Build history of the part. All positions in model axes, mm. Face numbers are marked on the shaded views. A direction names the side the tool comes from. Coordinates: 2 decimals unless noted, no trailing zeros. Loops run counter-clockwise (first coordinate to the right, second up) from the corner with the lowest first, then second, coordinate; pieces in that order, holes last.
Item 1: Cut at C-C (x = 109.5). List the corners of the cut face in (y, z).
Item 2: Drill centre lines: line 1 along X through (y, z) = (49, -20.5); line 2 along Z through (x, y) = (-56, 8.5); line 3 along X through (y, z) = (37, 3.5). Where is each one in solid material? Low to high.
Item 3: 3-axis set-ups, long thin cutter, end or side, ignore diameter. For the marked faces 1, 2, 3 and 4: which of +Z, -Z, +X, -X, +Y, -Y reach the whole face in a straight line?
Item 4: Flat gauge pins, fed straight in: pin 1 (2.5 mm diameter, centred on x = -20.5, y = 47, fed in from -Z); pin 2 (2 mm diameter, centred on x = -50.5, y = 40, fed in from +Z); pin 3 (2 mm diameter, centred on y = 32, z = 4.5, fed in from -X). Where does each tip first touch, or does it go through?
Item 5: Cut at A-A (y = 12). List the corners of the cut face in (x, z).
Item 6: Cut at B-B (z = 21). List the corners of the cut face in (x, y), and give its area (3 significant figures).
Item 7: Mould opens along Z. For the marked faces 5, 6 and 7 say: released by +Z, released by -Z, zero draft, split by the parting line, or undercut.
Item 8: Cut at D-D (z = -25). List the corners of the cut face in (x, y), and give its area (4 significant figures).
from build123d import *

# Parameters (mm, degrees)
BOSS_EXTRUDE1_DEPTH             = 135
BOSS_EXTRUDE2_REACH             = 151.416
BOSS_EXTRUDE2_DIRECTION_2_REACH = 151.416
CUT_EXTRUDE1_DEPTH              = 50
BOSS_EXTRUDE3_DEPTH             = 50
SKETCH9_R                       = 2
CUT_EXTRUDE2_DEPTH              = 262.164206304
CUT_EXTRUDE3_START              = -2
SKETCH10_W                      = 8.681737756
SKETCH10_H                      = 10
CUT_EXTRUDE3_DEPTH              = 260.164206304
SKETCH11_W                      = 78.8
SKETCH11_H                      = 50
SKETCH11_W_2                    = 40.4
BOSS_EXTRUDE4_DEPTH             = 2
BOSS_EXTRUDE5_DEPTH             = 131.8


with BuildPart() as part:
    # Sketch1 → Boss-Extrude1 (new, symmetric)
    with BuildSketch(Plane(origin=(0, 0, 0), x_dir=(0, 0, -1), z_dir=(1, 0, 0))):
        Polygon((0, 0), (0, 53), (-3, 53), (-3, 3), (-40, 3), (-40, 0), (-40, -17), (-30, -17), (-30, -5), (-25, 0), align=None)
    extrude(amount=BOSS_EXTRUDE1_DEPTH, both=True)

    # Sketch2 → Cut-Revolve1 (revolve, cut)
    with BuildSketch(Plane(origin=(0, 0, 0), x_dir=(0, 0, -1), z_dir=(1, 0, 0))):
        Polygon((-66, 3), (-30, 3), (-39, -112), (-66, -112), align=None)
    revolve(axis=Axis((0, 3, 66), (0, -1, 0)), mode=Mode.SUBTRACT)

    # Sketch3 → Cut-Revolve2 (revolve, cut)
    with BuildSketch(Plane(origin=(75, 0, 0), x_dir=(0, 0, -1), z_dir=(1, 0, 0))):
        Polygon((-30, 3), (-66, 3), (-66, -112), (-39, -112), align=None)
    cut_revolve2 = revolve(axis=Axis((75, 3, 66), (0, -1, 0)), mode=Mode.SUBTRACT)

    # Sketch4 → Cut-Revolve3 (revolve, cut)
    with BuildSketch(Plane(origin=(150, 0, 0), x_dir=(0, 0, -1), z_dir=(1, 0, 0))):
        Polygon((-30, 3), (-66, 3), (-66, -112), (-39, -112), align=None)
    cut_revolve3 = revolve(axis=Axis((150, 3, 66), (0, -1, 0)), mode=Mode.SUBTRACT)

    # Boss-Extrude2: up to this face of the body (flat: up to its plane)
    boss_extrude2_end = Plane(part.part.faces().sort_by_distance((0, 53, 1.5))[0])
    # Sketch5 → Boss-Extrude2 (add, up to the picked face)
    with BuildSketch(Plane(origin=(0, 3, 0), x_dir=(1, 0, 0), z_dir=(0, 1, 0)), mode=Mode.PRIVATE) as boss_extrude2_sk1:
        Polygon((89.696341704, -3), (135, -3), (135, 27.780279129), (135, 31.407195461), (84.358099725, -3), align=None)
    boss_extrude2_tool1 = split(extrude(boss_extrude2_sk1.sketch, amount=BOSS_EXTRUDE2_REACH, mode=Mode.PRIVATE), bisect_by=boss_extrude2_end, keep=Keep.BOTH, mode=Mode.PRIVATE)
    boss_extrude2 = boss_extrude2_tool1.solids().sort_by(Axis((118.119367, 3, -8.469065), (0, 1, 0)))[0]
    add(boss_extrude2)

    # Boss-Extrude2 direction 2: up to this face of the body (flat: up to its plane)
    boss_extrude2_direction_2_end = Plane(part.part.faces().sort_by_distance((0, 0, 12.5))[0])
    # Sketch5 → Boss-Extrude2 direction 2 (add, up to the picked face)
    with BuildSketch(Plane(origin=(0, 3, 0), x_dir=(1, 0, 0), z_dir=(0, 1, 0)), mode=Mode.PRIVATE) as boss_extrude2_direction_2_sk1:
        Polygon((89.696341704, -3), (135, -3), (135, 27.780279129), (135, 31.407195461), (84.358099725, -3), align=None)
    boss_extrude2_direction_2_tool1 = split(extrude(boss_extrude2_direction_2_sk1.sketch, amount=-BOSS_EXTRUDE2_DIRECTION_2_REACH, mode=Mode.PRIVATE), bisect_by=boss_extrude2_direction_2_end, keep=Keep.BOTH, mode=Mode.PRIVATE)
    boss_extrude2_direction_2 = boss_extrude2_direction_2_tool1.solids().sort_by(Axis((118.119367, 3, -8.469065), (0, -1, 0)))[0]
    add(boss_extrude2_direction_2)

    # Sketch7 → Cut-Extrude1 (cut)
    with BuildSketch(Plane(origin=(0, 3, 0), x_dir=(1, 0, 0), z_dir=(0, 1, 0))):
        Polygon((89.696341704, -3), (135, 27.780279129), (135, -3), align=None)
    cut_extrude1 = extrude(amount=CUT_EXTRUDE1_DEPTH, mode=Mode.SUBTRACT)

    # Sketch8 → Boss-Extrude3 (add)
    with BuildSketch(Plane(origin=(0, 3, 0), x_dir=(1, 0, 0), z_dir=(0, 1, 0))):
        Polygon((135, 27.780279129), (127.311099154, 22.556274642), (135, 11.239439757), align=None)
    boss_extrude3 = extrude(amount=BOSS_EXTRUDE3_DEPTH)

    # Sketch9 → Cut-Extrude2 (cut, through all)
    with BuildSketch(Plane(origin=(97.588254801, 0, -66.303557715), x_dir=(0.5619827673392628, 0, 0.8271489401635621), z_dir=(-0.8271489401635621, 0, 0.5619827673392628))):
        with Locations((62.889245152, 33)):
            Circle(SKETCH9_R)
    cut_extrude2 = extrude(amount=-CUT_EXTRUDE2_DEPTH, mode=Mode.SUBTRACT)

    # Sketch10 → Cut-Extrude3 (cut, through all)
    with BuildSketch(Plane(origin=(97.588254801, 0, -66.303557715), x_dir=(0.5619827673392628, 0, 0.8271489401635621), z_dir=(-0.8271489401635621, 0, 0.5619827673392628)).offset(CUT_EXTRUDE3_START)):
        with Locations((62.23011403, 33)):
            Rectangle(SKETCH10_W, SKETCH10_H)
    cut_extrude3 = extrude(amount=-CUT_EXTRUDE3_DEPTH, mode=Mode.SUBTRACT)

    # Mirror1: Cut-Revolve2, Cut-Revolve3, Boss-Extrude2, Boss-Extrude2 direction 2, Cut-Extrude1, Boss-Extrude3, Cut-Extrude2, Cut-Extrude3 across plane
    add(cut_revolve2.mirror(Plane(origin=(0, 0, 0), x_dir=(0, 0, 1), z_dir=(1, 0, 0))), mode=Mode.SUBTRACT)
    add(cut_revolve3.mirror(Plane(origin=(0, 0, 0), x_dir=(0, 0, 1), z_dir=(1, 0, 0))), mode=Mode.SUBTRACT)
    add(boss_extrude2.mirror(Plane(origin=(0, 0, 0), x_dir=(0, 0, 1), z_dir=(1, 0, 0))))
    add(boss_extrude2_direction_2.mirror(Plane(origin=(0, 0, 0), x_dir=(0, 0, 1), z_dir=(1, 0, 0))))
    add(cut_extrude1.mirror(Plane(origin=(0, 0, 0), x_dir=(0, 0, 1), z_dir=(1, 0, 0))), mode=Mode.SUBTRACT)
    add(boss_extrude3.mirror(Plane(origin=(0, 0, 0), x_dir=(0, 0, 1), z_dir=(1, 0, 0))))
    add(cut_extrude2.mirror(Plane(origin=(0, 0, 0), x_dir=(0, 0, 1), z_dir=(1, 0, 0))), mode=Mode.SUBTRACT)
    add(cut_extrude3.mirror(Plane(origin=(0, 0, 0), x_dir=(0, 0, 1), z_dir=(1, 0, 0))), mode=Mode.SUBTRACT)

    # Sketch11 → Boss-Extrude4 (add)
    with BuildSketch(Plane.XY.offset(3)):
        with Locations((-26.5, 28)):
            Rectangle(SKETCH11_W, SKETCH11_H)
        with Locations((45.7, 28)):
            Rectangle(SKETCH11_W_2, SKETCH11_H)
    extrude(amount=BOSS_EXTRUDE4_DEPTH)

    # Sketch12 → Boss-Extrude5 (add)
    with BuildSketch(Plane.ZY.offset(65.9)):
        with BuildLine():
            Line((6, 53), (6, 45))
            ThreePointArc((6, 45), (6.585786438, 43.585786438), (8, 43))
            Line((8, 43), (25, 43))
            Line((25, 43), (25, 3))
            Line((25, 3), (26, 3))
            Line((26, 3), (26, 43))
            ThreePointArc((26, 43), (25.707106781, 43.707106781), (25, 44))
            Line((25, 44), (8, 44))
            ThreePointArc((8, 44), (7.292893219, 44.292893219), (7, 45))
            Line((7, 45), (7, 53))
            Line((7, 53), (6, 53))
        make_face()
    extrude(amount=-BOSS_EXTRUDE5_DEPTH)


solid = part.part
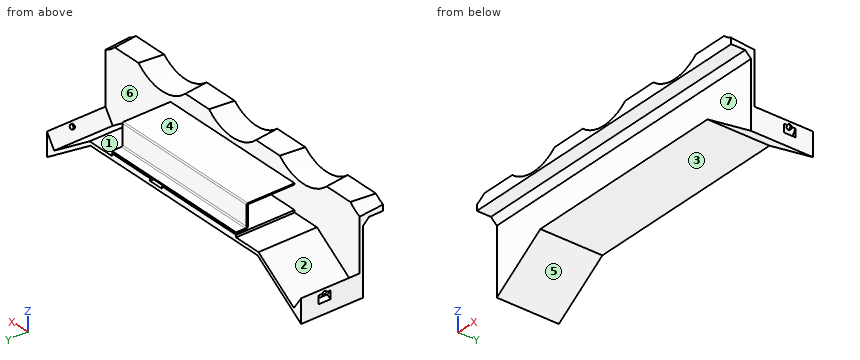
Filled sheet:
1. outline: (-17, 30) - (-5, 30) - (0, 25) - (0, -14.08) - (53, -14.08) - (53, -10.46) - (3, -10.46) - (3, 40) - (-17, 40) - close
2. line 1: x = -135 to -128.71, -124.28 to -118.95, 118.95 to 124.28, 128.71 to 135
2. line 2: z = 0 to 5, 25 to 26
2. line 3: x = -65.9 to 12.9, 25.5 to 65.9
3. face 1: +Z, +X, +Y
3. face 2: +Z, +Y
3. face 3: -Z, +Y, -Y
3. face 4: +Z, +X, -X, +Y
4. pin 1: stops at z = 0
4. pin 2: stops at z = 26
4. pin 3: stops at x = -65.9
5. outline: (-135, -31.41) - (-88.77, 0) - (88.77, 0) - (135, -31.41) - (135, -11.24) - (127.31, -22.56) - (89.7, 3) - (65.9, 3) - (65.9, 5) - (25.5, 5) - (25.5, 3) - (12.9, 3) - (12.9, 5) - (-65.9, 5) - (-65.9, 3) - (-89.7, 3) - (-127.31, -22.56) - (-135, -11.24) - close; (-65.9, 25) - (65.9, 25) - (65.9, 26) - (-65.9, 26) - close
6. outline: (-135, 0) - (135, 0) - (135, 3) - (-135, 3) - close; (-65.9, 43) - (65.9, 43) - (65.9, 44) - (-65.9, 44) - close
6. area: 942 mm2
7. face 5: released by -Z
7. face 6: undercut
7. face 7: zero draft
8. outline: (-135, 0) - (-125.57, 0) - (-125.57, 53) - (-135, 53) - close; (125.57, 0) - (135, 0) - (135, 53) - (125.57, 53) - close
8. area: 1,000 mm2
